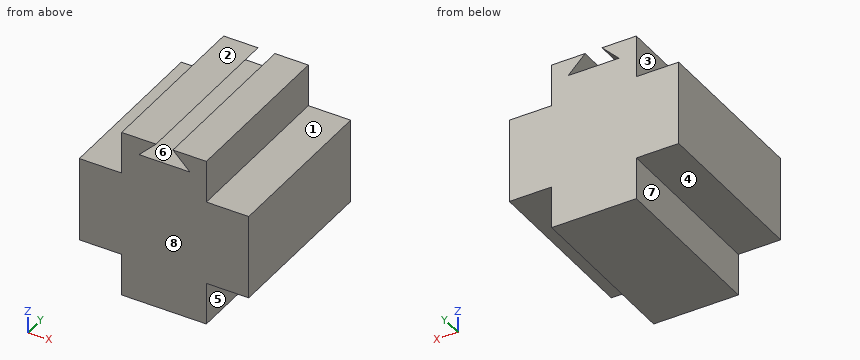
Autodesk Inventor part; units mm, degrees
ref_plane "YZ Plane" through (0, 0, 0) normal (1, 0, 0) x (0, 1, 0)
ref_plane "XZ Plane" through (0, 0, 0) normal (0, 1, 0) x (-1, 0, 0)
ref_plane "XY Plane" through (0, 0, 0) normal (0, 0, 1) x (1, 0, 0)
sketch "Sketch1" plane through (0, 0, 0) normal (0, 1, 0) x (-1, 0, 0)
  line L0 (-25.4, -12.7) -> (25.4, -12.7)
  line L1 (25.4, -12.7) -> (25.4, 12.7)
  line L2 (25.4, 12.7) -> (-25.4, 12.7)
  line L3 (-25.4, 12.7) -> (-25.4, -12.7)
  line L4 (-25.4, -12.7) -> (25.4, 12.7) construction
  line L5 (25.4, -12.7) -> (-25.4, 12.7) construction
  point P0 (0, 0)
  dimension "d0" = 25.4
  dimension "d1" = 50.8
extrude "Extrusion1" add sketch "Sketch1" along normal mid plane 50.8
sketch "Sketch2" plane through (-25.4, 25.4, 12.7) normal (0, 0, 1) x (1, 0, 0)
  line L0 (50.8, 0) -> (0, 0)
  line L1 (38.1, -50.8) -> (12.7, -50.8)
  line L2 (12.7, -50.8) -> (12.7, 0)
  line L3 (12.7, 0) -> (38.1, 0)
  line L4 (38.1, 0) -> (38.1, -50.8)
  line L5 (38.1, -50.8) -> (12.7, 0) construction
  line L6 (12.7, -50.8) -> (38.1, 0) construction
  point P0 (25.4, -25.4)
  dimension "d4" = 50.8
  dimension "d5" = 25.4
extrude "Extrusion2" add sketch "Sketch2" along normal blind 12.7 and the other way blind 38.1
sketch "Sketch3" plane through (0, -25.4, 0) normal (0, -1, 0) x (1, 0, 0)
  line L0 (12.7, 25.4) -> (-12.7, 25.4)
  line L1 (0, 25.4) -> (-2.4016, 25.4)
  line L2 (-7.4816, 20.32) -> (7.7584, 20.32)
  line L3 (7.7584, 20.32) -> (2.6784, 25.4)
  line L4 (-2.4016, 25.4) -> (-7.4816, 20.32)
  point P0 (0, 0)
  dimension "d10" = 5.08
  dimension "d11" = 5.08
  dimension "d12" = 15.24
  dimension "d13" = 45
  dimension "d14" = 25.4
  dimension "d15" = 45
extrude "Extrusion3" cut sketch "Sketch3" against normal up to next
properties part number "test3"
Verification items for the finished model (mm, model axes). Face numbers are marked on the shaded views. A direction names the side the tool comes from. Give positions to 0.01 mm unless a question says otherwise; leave off trailing zeros. Loops run counter-clockwise (first coordinate to the right, second up) from the corner with the lowest first, then second, coordinate; pieces in that order, holes last. Notation, with made-up numbers: M 33,-20 L 52,-20 A35 cw 52,14 Z; hole C -40,-20.5 d8. An arc over 180 degrees is marked long. One line per question, with ' | ' between items.
Item 1: Section check C-C, the plane z = 17.5. Record the cut outline in (x, y).
Completed:
outline: M -12.7,-25.4 L 12.7,-25.4 L 12.7,25.4 L -12.7,25.4 Z
Item 2: Section check B-B, the plane y = 14.5. Record the cut outline in (x, z).
Completed:
outline: M -25.4,-12.7 L -12.7,-12.7 L -12.7,-25.4 L 12.7,-25.4 L 12.7,-12.7 L 25.4,-12.7 L 25.4,12.7 L 12.7,12.7 L 12.7,25.4 L 2.68,25.4 L 7.76,20.32 L -7.48,20.32 L -2.4,25.4 L -12.7,25.4 L -12.7,12.7 L -25.4,12.7 Z
Item 3: Section check A-A, the plane x = 4. Record the cut outline in (y, z).
Completed:
outline: M -25.4,-25.4 L 25.4,-25.4 L 25.4,20.32 L -25.4,20.32 Z; M -25.4,24.08 L 25.4,24.08 L 25.4,25.4 L -25.4,25.4 Z
Item 4: Thickness scan on line 1 (Z direction, x = -18.5, y = -16.5); line 2 (Z direction, x = 2, y = 12.5); line 3 (Z direction, x = 4, y = -8). Record the ranges inside material, lowest first. Write a range as [from, to].
Completed:
line 1: z = [-12.7, 12.7] | line 2: z = [-25.4, 20.32] | line 3: z = [-25.4, 20.32], [24.08, 25.4]
Item 5: Draft check along X on the marked faces 6, 7 and 8. Enter one of: +X half, -X half, draft (parallel to the pull), parting line (faces both ways), or undercut.
Completed:
face 6: undercut | face 7: -X half | face 8: draft
Item 6: Tool access check on the marked faces 1, 2, 3, 4 and 5. Record the directions out of +Z, -Z, +X, -X, +Y, -Y that give a thin tool (end or side, any length) a straight path to the whole face; none if there is none.
Completed:
face 1: +Z, +X, +Y, -Y | face 2: +Z, +X, -X, +Y, -Y | face 3: +Z, -X, +Y, -Y | face 4: -Z, -X, +Y, -Y | face 5: -Z, +X, +Y, -Y
Item 7: Section check D-D, the plane x = -6. Record the cut outline in (y, z).
Completed:
outline: M -25.4,-25.4 L 25.4,-25.4 L 25.4,20.32 L -25.4,20.32 Z; M -25.4,21.8 L 25.4,21.8 L 25.4,25.4 L -25.4,25.4 Z
Item 8: Depth check by flat-ended pin: P1, Ø3, axis at x = -16.5, y = -6.5, coming from the +Z side; P2, Ø6.5, axis at x = 18, y = -12.5, coming from the -Z side; P3, Ø6.5, axis at y = 6.5, z = -21.5, coming from the +X side. Enter the tip coordinate at first touch or a pass-through.
Completed:
P1: stops at z = 12.7 | P2: stops at z = -12.7 | P3: stops at x = 12.7
